Design review of the part built by this model. Coordinates are the model's own, in mm. A direction names the side the tool comes from. Coordinates: 2 decimals unless noted, no trailing zeros. Loops run counter-clockwise (first coordinate to the right, second up) from the corner with the lowest first, then second, coordinate; pieces in that order, holes last. Notation, with made-up numbers: M 24.5,82 L 59.5,82 A32 ccw 59.5,114 Z; hole C -26,-7 d11. An arc over 180 degrees is marked long. Answer as a JSON object with one key per item and string values. Group by question number.
1. Consider section B-B (y = 20). State the section outline as (x, z) points.
2. Consider section A-A (x = 37). State the section outline as (y, z) points, then the cut area to 3 significant figures.
3. Consider section C-C (x = 19). State the section outline as (y, z) points, then the cut area to 3 significant figures.
4. Draft analysis for pull direction Z (two halves, no side actions). For faces 1 (the flat face through (15, 27, 9)), 2 (the flat face through (21, 9, 0)), 3 (the flat face through (12, 20, 7)), state which applies: +Z half, -Z half, draft (parallel to the pull), parting line (faces both ways), or undercut.
5. Insertion check: pin 1 (7 mm diameter, centred on y = 22, z = 6, fed in from -X); pin 2 (6 mm diameter, centred on x = 10.5, y = 20.5, fed in from +Z); pin 3 (6 mm diameter, centred on x = 36, z = 8.5, fed in from +Y); pin 4 (1 mm diameter, centred on y = 14.5, z = 5, fed in from +X). Each pin has a flat end and moves straight along its axis. Give the tip position at first contact, or say it passes through.
6. Machinability: for faces 4 (the cylindrical face through (13.479, 31.724, 6.544)), 5 (the flat face through (33, 6, 7)), 6 (the flat face through (20, 31, 7)), 7 (the flat face through (26, 32.8, 7)), which of the approach directions +Z, -Z, +X, -X, +Y, -Y give a long, thin tool a straight path to every point of the face, cutting with its end or side? Answer none if there is none.
7. To check wall thickness, follow probe 1 along X at (y, z) = (2.9, 7); probe 2 along X at (y, z) = (31, 7); probe 3 along Y at (x, z) = (13.15, 7). State the ranges of each line that lie inside material, in increasing order.
8. Consider section D-D (z = 7). Count the separate pieces of the cut face and the enclosed holes in it, then the cut area to 3 significant figures.
from build123d import *

# Parameters (mm, degrees)
BOSS_EXTRUDE1_DEPTH = 14
SKETCH2_R           = 2.75
CUT_EXTRUDE1_DEPTH  = 7
SKETCH3_R           = 2
CUT_EXTRUDE2_DEPTH  = 31
SKETCH4_R           = 3.5
CUT_EXTRUDE3_DEPTH  = 3


with BuildPart() as part:
    # Sketch1 → Boss-Extrude1 (new body)
    with BuildSketch(Plane.XY):
        with BuildLine():
            Line((0, 0), (42, 0))
            Line((42, 0), (42, 6))
            Line((42, 6), (30, 6))
            Line((30, 6), (30, 32.8))
            Line((30, 32.8), (22, 32.8))
            Line((22, 32.8), (22, 24.898979486))
            ThreePointArc((22, 24.898979486), (21, 15), (20, 24.898979486))
            Line((20, 24.898979486), (20, 32.8))
            Line((20, 32.8), (12, 32.8))
            Line((12, 32.8), (12, 6))
            Line((12, 6), (0, 6))
            Line((0, 6), (0, 0))
        make_face()
    extrude(amount=BOSS_EXTRUDE1_DEPTH)

    # Sketch2 → Cut-Extrude1 (cut, through all)
    with BuildSketch(Plane(origin=(0, 6, 0), x_dir=(1, 0, 0), z_dir=(0, 1, 0))):
        with Locations((5, -7)):
            Circle(SKETCH2_R)
        with Locations((37, -7)):
            Circle(SKETCH2_R)
    extrude(amount=-CUT_EXTRUDE1_DEPTH, mode=Mode.SUBTRACT)

    # Sketch3 → Cut-Extrude2 (cut, through all)
    with BuildSketch(Plane.ZY.offset(-12)):
        with Locations((7, 28.254234055)):
            Circle(SKETCH3_R)
    extrude(amount=-CUT_EXTRUDE2_DEPTH, mode=Mode.SUBTRACT)

    # Sketch4 → Cut-Extrude3 (cut)
    with BuildSketch(Plane.ZY.offset(-12)):
        with Locations((7, 28.254234055)):
            Circle(SKETCH4_R)
    extrude(amount=-CUT_EXTRUDE3_DEPTH, mode=Mode.SUBTRACT)


solid = part.part
Findings below:
{
 "1": {"outline": "M 12,0 L 16,0 L 16,14 L 12,14 Z; M 26,0 L 30,0 L 30,14 L 26,14 Z"},
 "2": {"outline": "M 0,0 L 6,0 L 6,4.25 L 0,4.25 Z; M 0,9.75 L 6,9.75 L 6,14 L 0,14 Z", "area": "51.0 mm^2"},
 "3": {"outline": "M 0,0 L 15.42,0 L 15.42,14 L 0,14 Z; M 24.58,0 L 32.8,0 L 32.8,14 L 24.58,14 Z; hole C 28.25,7 d4", "area": "318 mm^2"},
 "4": {"face 1": "undercut", "face 2": "-Z half", "face 3": "draft"},
 "5": {"pin 1": "stops at x = 12", "pin 2": "stops at z = 14", "pin 3": "stops at y = 6", "pin 4": "stops at x = 30"},
 "6": {"face 4": "-X", "face 5": "+Z, -Z, +X, +Y", "face 6": "+Z, -Z, +Y", "face 7": "+Z, -Z, +X, -X, +Y"},
 "7": {"probe 1": "x = 0 to 2.25, 7.75 to 34.25, 39.75 to 42", "probe 2": "x = 15 to 20, 22 to 30", "probe 3": "y = 0 to 24.75, 31.75 to 32.8"},
 "8": {"separate pieces": "5", "enclosed holes": "0", "area": "501 mm^2"}
}
